Drawing for the job (mm, zero at the part's lowest x, y, z). A direction names the side the tool comes from. Give positions to 0.01 mm unless a question says otherwise; leave off trailing zeros. Write each loop counter-clockwise with the first axis right and the second up, starting at its lowest first coordinate (ties: lowest second). Pieces come first, ordered by that corner, then holes.
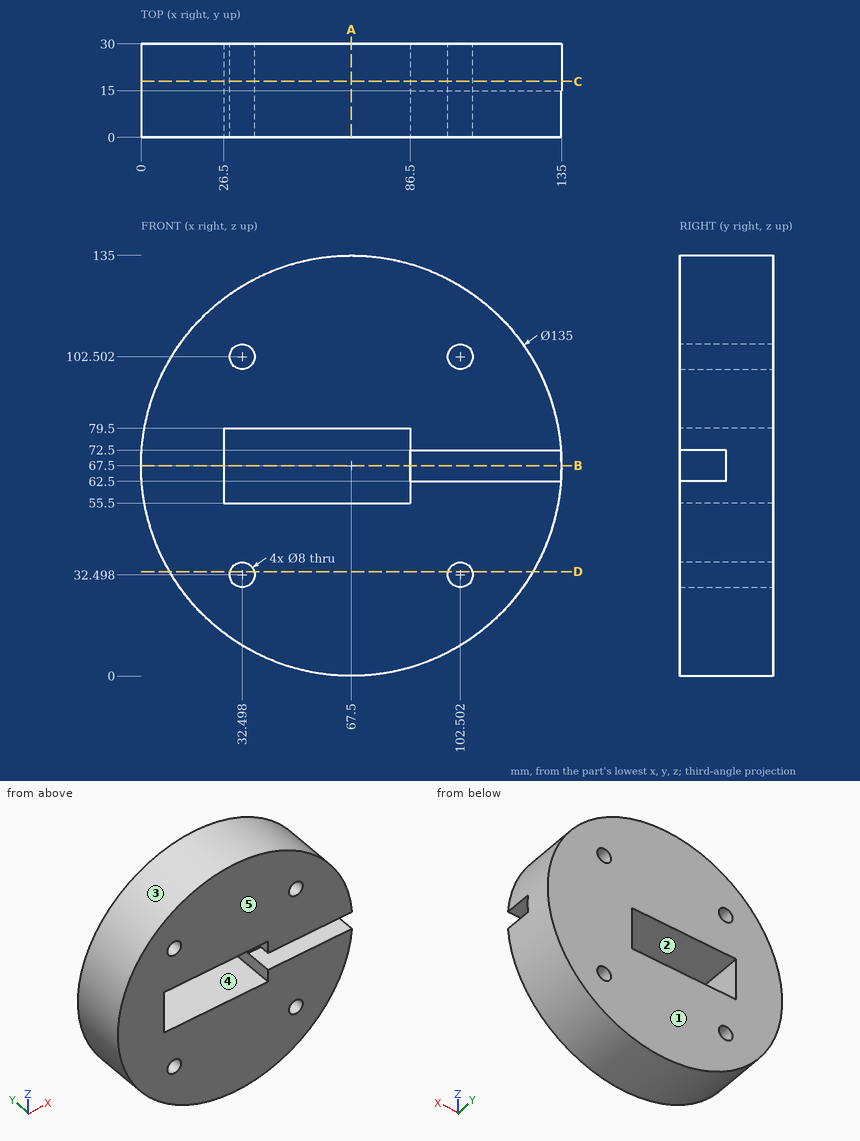
1. Slice it at A-A, the plane x = 67.5. Write the cut outline in (y, z), and give its area (3 significant figures).
Calculated:
outline: (0, 0) - (30, 0) - (30, 55.5) - (0, 55.5) - close; (0, 79.5) - (30, 79.5) - (30, 135) - (0, 135) - close
area: 3,330 mm2
2. Slice it at C-C, the plane y = 18. Write the cut outline in (x, z).
Calculated:
outline: circle Ø135 at (67.5, 67.5); hole (26.5, 55.5) - (86.5, 55.5) - (86.5, 79.5) - (26.5, 79.5) - close; hole circle Ø8 at (32.5, 32.5); hole circle Ø8 at (32.5, 102.5); hole circle Ø8 at (102.5, 32.5); hole circle Ø8 at (102.5, 102.5)
3. Which spindle directions (+Z, -Z, +X, -X, +Y, -Y) get a long thin tool onto all of the face, cutting with end or side? Do the marked faces 1 and 2. Say none if no direction does.
Calculated:
face 1: +Z, -Z, +X, -X, +Y
face 2: +Y, -Y
4. Pin check, flat tips, straight feed: P1, Ø12, axis at x = 83.5, y = 21, coming from the -Z side (3 decimals); P2, Ø2, axis at x = 16.5, y = 4, coming from the +Z side (1 decimal); P3, Ø4, axis at x = 100.5, y = 25, coming from the -Z side. Stop position of each tip, or through.
Calculated:
P1: stops at z = 0.745
P2: stops at z = 112.8
P3: stops at z = 7.54
5. Probe probe 1 along Z at (x, y) = (30.5, 22) (1 decimal); probe 2 along X at (y, z) = (4.5, 32); probe 3 along X at (y, z) = (16.25, 33). List the from-to ranges inside material, lowest first.
Calculated:
probe 1: z = 11 to 29, 36 to 55.5, 79.5 to 99, 106 to 124
probe 2: x = 10.09 to 28.53, 36.47 to 98.53, 106.47 to 124.91
probe 3: x = 9.48 to 28.53, 36.47 to 98.53, 106.47 to 125.52
6. Pull direction X, two halves, no side cores. Call the marked faces 3, 4 and 5: +X half, -X half, draft (parallel to the pull), parting line (faces both ways), or undercut.
Calculated:
face 3: parting line
face 4: undercut
face 5: draft
7. Slice it at B-B, the plane z = 67.5. Write the cut outline in (x, y).
Calculated:
outline: (0, 0) - (26.5, 0) - (26.5, 30) - (0, 30) - close; (86.5, 15) - (135, 15) - (135, 30) - (86.5, 30) - close
8. Slice it at D-D, the plane z = 33.5. Write the cut outline in (x, y).
Calculated:
outline: (9.19, 0) - (28.63, 0) - (28.63, 30) - (9.19, 30) - close; (36.37, 0) - (98.63, 0) - (98.63, 30) - (36.37, 30) - close; (106.37, 0) - (125.81, 0) - (125.81, 30) - (106.37, 30) - close
